The listing builds one solid part. Answer for the finished solid, in the listing's coordinates (mm). Face numbers are marked on the shaded views. A direction names the side the tool comes from. Round coordinates to 2 decimals unless told otherwise and drop trailing zeros. Write each loop counter-clockwise with the first axis right and the second up, starting at its lowest first coordinate (ties: lowest second). Pieces come first, ordered by that corner, then holes. Notation, with made-up numbers: (-2, -26.75) - (28, -26.75) arc R18 ccw to (28, -11.75) - close; hole circle Ø8 at (44.25, 41). An arc over 180 degrees is marked (long way). Answer in a Markdown table with one row per item.
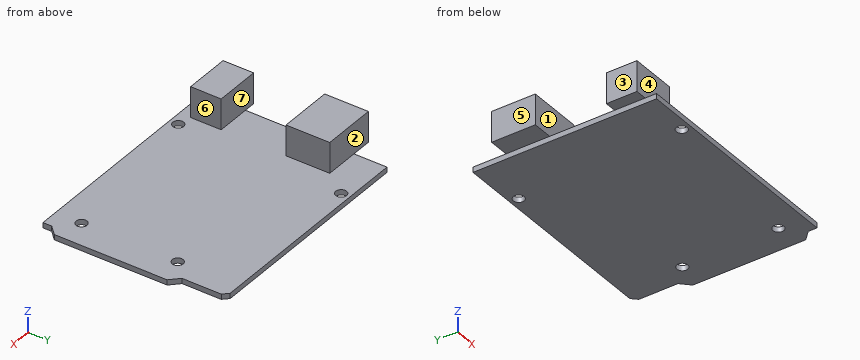
from build123d import *

# Parameters (mm, degrees)
F0_R     = 1.5875
F1_DEPTH = 1.524
F2_W     = 5.913735792
F2_H     = 12.7
F2_W_2   = 9.961264208
F2_W_3   = 3.373735792
F2_H_2   = 8.89
F3_DEPTH = 8.89


# Not quite as in the source:
# - a feature names something its author has since deleted; it is built from what else it names


with BuildPart() as f1:
    # F0 (on Top) → F1 (new body)
    with BuildSketch(Plane.XY):
        Polygon((0, 53.34), (0, 0), (66.04, 0), (66.04, 2.54), (68.58, 5.08), (68.58, 37.846), (66.04, 40.386), (66.04, 51.816), (64.516, 53.34), align=None)
        with Locations((13.97, 2.54)):
            Circle(F0_R, mode=Mode.SUBTRACT)
        with Locations((60.96, 7.62)):
            Circle(F0_R, mode=Mode.SUBTRACT)
        with Locations((15.24, 50.8)):
            Circle(F0_R, mode=Mode.SUBTRACT)
        with Locations((60.96, 35.56)):
            Circle(F0_R, mode=Mode.SUBTRACT)
    extrude(amount=-F1_DEPTH)

    # F2 (on face) → F3 (join)
    with BuildSketch(Plane.XY):
        with Locations((-2.956867896, 37.39)):
            Rectangle(F2_W, F2_H)
        with Locations((4.980632104, 37.39)):
            Rectangle(F2_W_2, F2_H)
        with Locations((-1.686867896, 7.745)):
            Rectangle(F2_W_3, F2_H_2)
        with Locations((4.980632104, 7.745)):
            Rectangle(F2_W_2, F2_H_2)
    extrude(amount=F3_DEPTH)


solid = f1.part
(1) Section A-A (y = 7.62) is taken. Give the vertices of the cut face in (x, z).
Checked values:
| item | result |
|---|---|
| outline | (-3.37, 0) - (0, 0) - (0, -1.52) - (59.37, -1.52) - (59.37, 0) - (9.96, 0) - (9.96, 8.89) - (-3.37, 8.89) - close; (62.55, -1.52) - (68.58, -1.52) - (68.58, 0) - (62.55, 0) - close |
(2) For a pull along Y with two mould halves and no side action, classify the marked faces 1, 2 and 3 as pulls with the +Y half, pulls with the -Y half, needs draft (parallel to the pull), parting line crosses it, or undercut.
Checked values:
| item | result |
|---|---|
| face 1 | undercut |
| face 2 | pulls with the +Y half |
| face 3 | needs draft |
(3) Section D-D (y = 50.8) is taken. Give the vertices of the cut face in (x, z).
Checked values:
| item | result |
|---|---|
| outline | (0, -1.52) - (13.65, -1.52) - (13.65, 0) - (0, 0) - close; (16.83, -1.52) - (66.04, -1.52) - (66.04, 0) - (16.83, 0) - close |
(4) For the marked faces 4, 5, 6 and 7, determine the directions among +Z, -Z, +X, -X, +Y, -Y from which every point of the face is accessible in a straight line to the end or side of a thin tool.
Checked values:
| item | result |
|---|---|
| face 4 | +Z, +X, -X, -Y |
| face 5 | +Z, -Z, -X, +Y, -Y |
| face 6 | +Z, +X, +Y, -Y |
| face 7 | +Z, +X, -X |
(5) Section C-C (x = 60.96) is taken. Give the vertices of the cut face in (y, z).
Checked values:
| item | result |
|---|---|
| outline | (0, -1.52) - (6.03, -1.52) - (6.03, 0) - (0, 0) - close; (9.21, -1.52) - (33.97, -1.52) - (33.97, 0) - (9.21, 0) - close; (37.15, -1.52) - (53.34, -1.52) - (53.34, 0) - (37.15, 0) - close |
(6) Flat-ended cylindrical pins translate along their axes: pin 1 (4 mm diameter, centred on x = 15.24, y = 50.8, fed in from +Z); pin 2 (2.5 mm diameter, centred on x = 5, z = 3.5, fed in from +Y); pin 3 (1.9 mm diameter, centred on x = 60.96, y = 35.56, fed in from +Z); pin 4 (1.7 mm diameter, centred on y = 44, z = -0.5, fed in from +X). Find the tip coordinate at first contact, or state that the pin passes through.
Checked values:
| item | result |
|---|---|
| pin 1 | stops at z = 0 |
| pin 2 | stops at y = 43.74 |
| pin 3 | passes through |
| pin 4 | stops at x = 66.04 |
(7) Section B-B (z = 7) is taken. Give the vertices of the cut face in (x, y), and give its area (3 significant figures).
Checked values:
| item | result |
|---|---|
| outline | (-5.91, 31.04) - (9.96, 31.04) - (9.96, 43.74) - (-5.91, 43.74) - close; (-3.37, 3.3) - (9.96, 3.3) - (9.96, 12.19) - (-3.37, 12.19) - close |
| area | 320 mm2 |
(8) Find the intervals of material crossed by line 1 (Y direction, x = 60.96, z = -0.85); line 2 (Z direction, x = 45.5, y = 5); line 3 (X direction, y = 25.5, z = -0.25), in increasing order.
Checked values:
| item | result |
|---|---|
| line 1 | y = 0 to 6.03, 9.21 to 33.97, 37.15 to 53.34 |
| line 2 | z = -1.52 to 0 |
| line 3 | x = 0 to 68.58 |
